```python
from build123d import *

# Parameters (mm, degrees)
BOSS_EXTRUDE1_DEPTH        = 30
F_2_2_2_2_DIAMETER_HOLE1_D = 2.2


with BuildPart() as part:
    # Sketch1 → Boss-Extrude1 (new, symmetric)
    with BuildSketch(Plane.XY):
        with BuildLine():
            Line((-1.3, 0), (1.3, 0))
            ThreePointArc((1.3, 0), (2.826836794, 5.310885546), (6.941101056, 9))
            Line((6.941101056, 9), (6.941101056, 10))
            Line((6.941101056, 10), (-6.941101056, 10))
            Line((-6.941101056, 10), (-6.941101056, 9))
            ThreePointArc((-6.941101056, 9), (-2.826836794, 5.310885546), (-1.3, 0))
        make_face()
    extrude(amount=BOSS_EXTRUDE1_DEPTH, both=True)

    # Ø2.2 (2.2) Diameter Hole1 (through all)
    with Locations(Plane(origin=(0, 10, 15), x_dir=(0, 0, 1), z_dir=(0, 1, 0))):
        with Locations((0, 0), (-30, 0)):
            Hole(F_2_2_2_2_DIAMETER_HOLE1_D / 2)


solid = part.part
```
Read the model definition and answer for the solid it produces. Units are mm, in the model's axes. Give positions to 0.01 mm unless a question says otherwise; leave off trailing zeros. Write each loop counter-clockwise with the first axis right and the second up, starting at its lowest first coordinate (ties: lowest second). Pieces come first, ordered by that corner, then holes. Notation, with made-up numbers: (7.25, 88) -> (35.25, 88) arc R23 ccw to (35.25, 119) -> close; hole circle Ø6 at (68.5, 55.25). An arc over 180 degrees is marked (long way). Answer as a JSON object with one key per item and string values.
1) Straight lines are drawn through the part: probe 1 along Z at (x, y) = (-0.25, 7.5); probe 2 along Z at (x, y) = (0.75, 4.5); probe 3 along X at (y, z) = (8, -15). For each, find the intervals that lie inside material, in ascending order. Write a range as from..to.
Findings below:
{"probe 1": "z = -30..-16.07, -13.93..13.93, 16.07..30", "probe 2": "z = -30..-15.8, -14.2..14.2, 15.8..30", "probe 3": "x = -5.3..-1.1, 1.1..5.3"}
2) Section D-D on x = -3.5 is taken. Write down the section's boundary in (y, z), then the cut area to 3 significant figures.
Findings below:
{"outline": "(6.26, -30) -> (10, -30) -> (10, 30) -> (6.26, 30) -> close", "area": "225 mm^2"}
3) Section C-C on z = 25 is taken. Write down the section's boundary in (x, y), then the cut area to 3 significant figures.
Findings below:
{"outline": "(-6.94, 9) arc R10 cw to (-1.3, 0) -> (1.3, 0) arc R10 cw to (6.94, 9) -> (6.94, 10) -> (-6.94, 10) -> close", "area": "66.1 mm^2"}
4) Flat-ended cylindrical pins translate along their axes: pin 1 Ø4 at (x, z) = (1, 1.5) entering from -Y; pin 2 Ø4 at (y, z) = (6.5, -14) entering from -X; pin 3 Ø4 at (y, z) = (2, 23) entering from +X. Find the tip coordinate at first contact, or state that the pin passes through.
Findings below:
{"pin 1": "stops at y = 0", "pin 2": "stops at x = -6.03", "pin 3": "stops at x = 2.13"}
5) Section B-B on y = 6 is taken. Write down the section's boundary in (x, z).
Findings below:
{"outline": "(-3.3, -30) -> (3.3, -30) -> (3.3, 30) -> (-3.3, 30) -> close; hole circle Ø2.2 at (0, -15); hole circle Ø2.2 at (0, 15)"}
6) Section A-A on z = -15 is taken. Write down the section's boundary in (x, y).
Findings below:
{"outline": "(-6.94, 9) arc R10 cw to (-1.3, 0) -> (-1.1, 0) -> (-1.1, 10) -> (-6.94, 10) -> close; (1.1, 0) -> (1.3, 0) arc R10 cw to (6.94, 9) -> (6.94, 10) -> (1.1, 10) -> close"}
7) For a pull along Z with two mould halves and no side action, classify faces 1 (the flat face through (0, 6, 30)), 2 (the flat face through (0, 0, 0)), 3 (the cylindrical face through (0, 4.9, 16.1)) as pulls with the +Z half, pulls with the -Z half, needs draft (parallel to the pull), parting line crosses it, or undercut.
Findings below:
{"face 1": "pulls with the +Z half", "face 2": "needs draft", "face 3": "undercut"}
